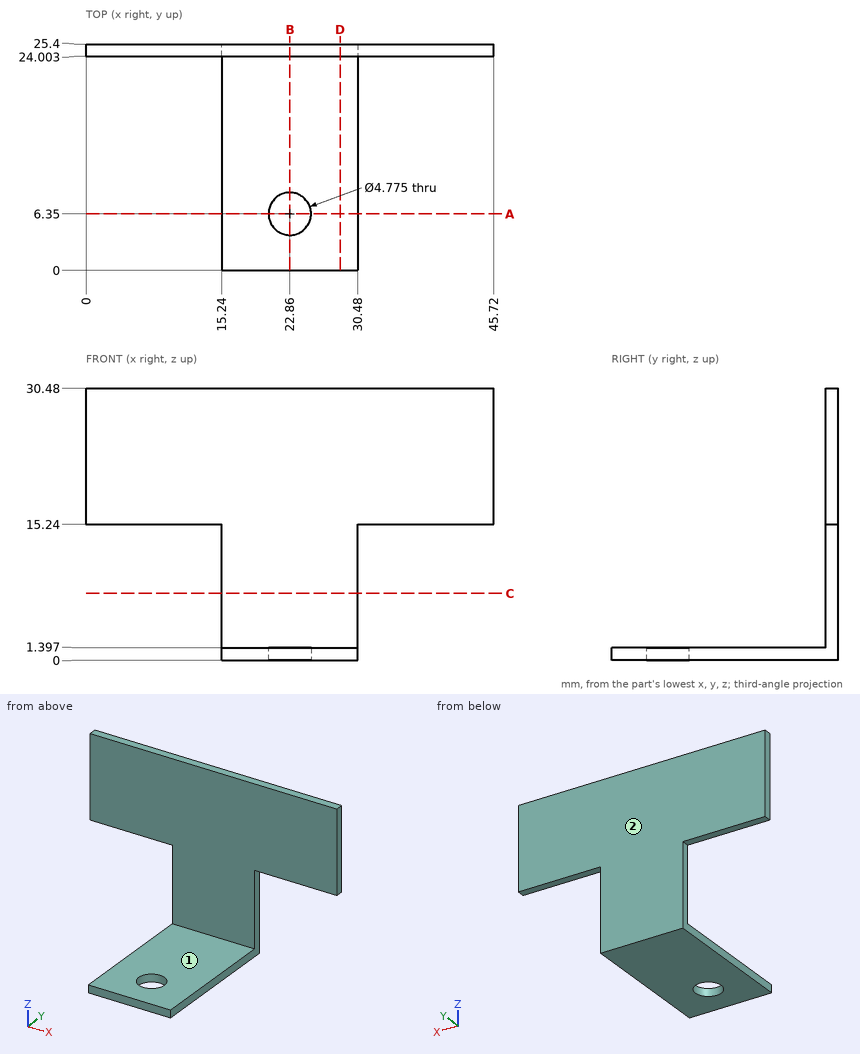
Source: three-view drawing plus pictorial views. Frame: mm from the lowest corner of the part. A direction names the side the tool comes from. Give positions to 0.01 mm unless a question says otherwise; leave off trailing zeros. Loops run counter-clockwise (first coordinate to the right, second up) from the corner with the lowest first, then second, coordinate; pieces in that order, holes last.
1) Section query A-A on y = 6.35. Return the cut outline in (x, z).
A:
outline: (15.24, 0) - (20.47, 0) - (20.47, 1.4) - (15.24, 1.4) - close; (25.25, 0) - (30.48, 0) - (30.48, 1.4) - (25.25, 1.4) - close
2) Section query B-B on x = 22.86. Return the cut outline in (y, z).
A:
outline: (0, 0) - (3.96, 0) - (3.96, 1.4) - (0, 1.4) - close; (8.74, 0) - (25.4, 0) - (25.4, 30.48) - (24, 30.48) - (24, 1.4) - (8.74, 1.4) - close
3) Contact query for flat-ended pins moving along their axis: pin 1 (7.5 mm diameter, centred on y = 12, z = 6.5, fed in from +X); pin 2 (12 mm diameter, centred on y = 13.5, z = 6.5, fed in from +X); pin 3 (1.5 mm diameter, centred on x = 10, y = 25, fed in from -Z); pin 4 (8 mm diameter, centred on x = 17, z = 13.5, fed in from -Y). Output: stop coordinate, or through.
A:
pin 1: passes through
pin 2: stops at x = 30.48
pin 3: stops at z = 15.24
pin 4: stops at y = 24
4) Reachability of the marked faces 1 and 2 from +Z, -Z, +X, -X, +Y, -Y: full face, straight path, thin tool, end or side. Return the list, or none.
A:
face 1: +Z, +X, -X, -Y
face 2: +Z, -Z, +X, -X, +Y
5) Section query C-C on z = 7.5. Return the cut outline in (x, y).
A:
outline: (15.24, 24) - (30.48, 24) - (30.48, 25.4) - (15.24, 25.4) - close
6) Section query D-D on x = 28.5. Return the cut outline in (y, z).
A:
outline: (0, 0) - (25.4, 0) - (25.4, 30.48) - (24, 30.48) - (24, 1.4) - (0, 1.4) - close
7) Line query: L1, parallel to Y at x = 22.86, z = 0.75; L2, parallel to Y at x = 40, z = 22; L3, parallel to Z at x = 24, y = 10.25. Output: solid intervals per line, ascending.
A:
L1: y = 0 to 3.96, 8.74 to 25.4
L2: y = 24 to 25.4
L3: z = 0 to 1.4
